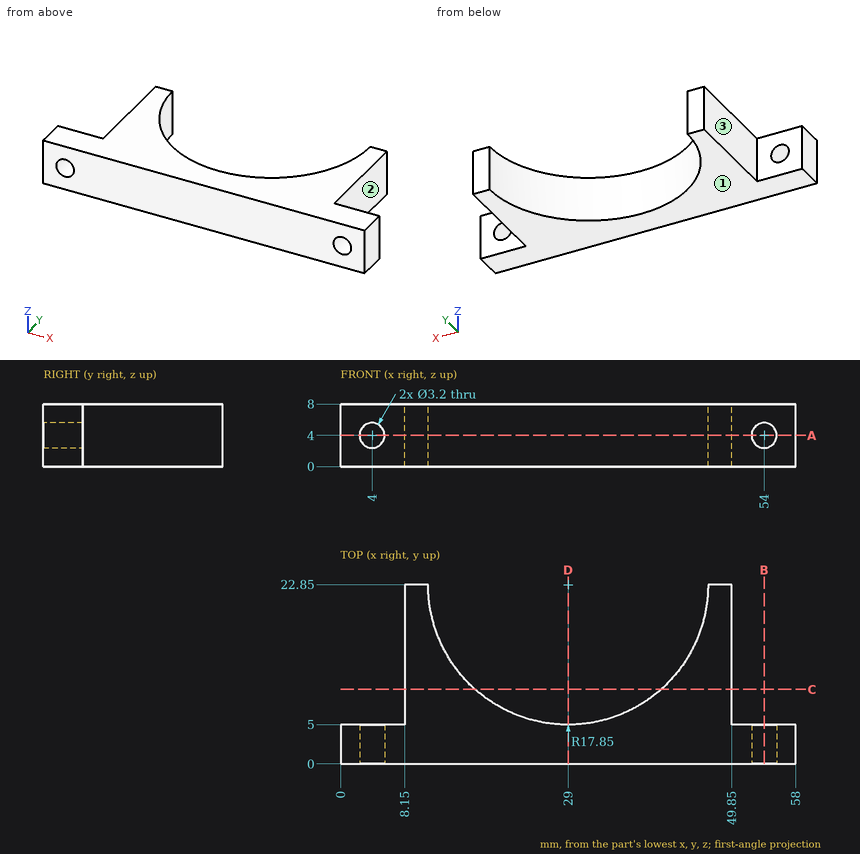
Input: dimensioned drawing with shaded views. Units: mm. Origin: part minimum x, y, z. A direction names the side the tool comes from. Round coordinates to 2 decimals unless told otherwise and drop trailing zeros. Loops run counter-clockwise (first coordinate to the right, second up) from the corner with the lowest first, then second, coordinate; pieces in that order, holes last. Notation, with made-up numbers: (60.25, 38.25) -> (113.25, 38.25) arc R24 cw to (113.25, 76.25) -> close; hole circle Ø7 at (47, 2). An arc over 180 degrees is marked (long way). Answer as a JSON object with one key per item and string values. Group by question number.
Q1. Section query C-C (y = 9.5). Output: boundary loops of the cut face in (x, z).
Q2. Ray query, line 1 (X direction, y = 2.2, z = 4); line 2 (X direction, y = 12.5, z = 1); line 3 (Y direction, x = 50, z = 1.5). Return the intervals inside material, ascending. Write a range as from..to.
Q3. Section query D-D (x = 29). Output: boundary loops of the cut face in (y, z).
Q4. Section query B-B (x = 54). Output: boundary loops of the cut face in (y, z), plus the area to 3 significant figures.
Q5. Access query for the marked faces 1, 2 and 3. Directions: +Z, -Z, +X, -X, +Y, -Y. A direction counts if a zero-diameter tool reaches every point of the face in a straight line with its end or side. Return the directions, or none.
Q6. Contact query for flat-ended pins moving along their axis: P1, Ø2, axis at x = 30, z = 3, coming from the -Y side; P2, Ø2.5, axis at x = 3, z = 2.5, coming from the +Y side; P3, Ø3, axis at x = 33, z = 3, coming from the +Y side; P4, Ø1, axis at x = 45.5, y = 20.5, coming from the +Z side. Output: stop coordinate, or through.
Q7. Section query A-A (z = 4). Output: boundary loops of the cut face in (x, y).
Completed:
{
 "1": {"outline": "(8.15, 0) -> (17.15, 0) -> (17.15, 8) -> (8.15, 8) -> close; (40.85, 0) -> (49.85, 0) -> (49.85, 8) -> (40.85, 8) -> close"},
 "2": {"line 1": "0..2.4, 5.6..52.4, 55.6..58", "line 2": "8.15..14.46, 43.54..49.85", "line 3": "0..5"},
 "3": {"outline": "(0, 0) -> (5, 0) -> (5, 8) -> (0, 8) -> close"},
 "4": {"outline": "(0, 0) -> (5, 0) -> (5, 2.4) -> (0, 2.4) -> close; (0, 5.6) -> (5, 5.6) -> (5, 8) -> (0, 8) -> close", "area": "24.0 mm²"},
 "5": {"face 1": "-Z, +X, -X, +Y, -Y", "face 2": "+Z, -Z, +X, +Y", "face 3": "+Z, -Z, -X, +Y"},
 "6": {"P1": "y = 0", "P2": "y = 5", "P3": "y = 5.87", "P4": "through"},
 "7": {"outline": "(0, 0) -> (2.4, 0) -> (2.4, 5) -> (0, 5) -> close; (5.6, 0) -> (52.4, 0) -> (52.4, 5) -> (49.85, 5) -> (49.85, 22.85) -> (46.85, 22.85) arc R17.85 cw to (11.15, 22.85) -> (8.15, 22.85) -> (8.15, 5) -> (5.6, 5) -> close; (55.6, 0) -> (58, 0) -> (58, 5) -> (55.6, 5) -> close"}
}
